```python
from build123d import *

# Parameters (mm, degrees)
SKETCH1_W               = 60
SKETCH1_H               = 160
BOSS_EXTRUDE1_DEPTH     = 3.175
M4_5_THROUGH_DEPTH      = 6.35
M4_5_THROUGH_DEPTH_BACK = 3.175
SKETCH3_R               = 2.75
SKETCH3_R_2             = 2.2
SKETCH4_R               = 1.3
M3_DRILL_DEPTH          = 8
SKETCH5_R               = 2.2
M4_THROUGH_DEPTH        = 6.35
SKETCH6_R               = 2.75
M5_THROUGH_DEPTH        = 6.35
SKETCH7_W               = 60
SKETCH7_H               = 30.2375
CUT_EXTRUDE1_DEPTH      = 6.35


with BuildPart() as part:
    # Sketch1 → Boss-Extrude1 (new, symmetric)
    with BuildSketch(Plane(origin=(0, 0, 0), x_dir=(1, 0, 0), z_dir=(0, 1, 0))):
        Rectangle(SKETCH1_W, SKETCH1_H)
    extrude(amount=BOSS_EXTRUDE1_DEPTH, both=True)

    # Sketch3 → M4/5_through (cut, two sides: drawn at the far end of the back side and taken through both)
    with BuildSketch(Plane(origin=(0, 0, 0), x_dir=(1, 0, 0), z_dir=(0, 1, 0)).offset(-M4_5_THROUGH_DEPTH_BACK)):
        with Locations(Location((20, 75.2375, 0), (0, 0, 270))):
            Circle(SKETCH3_R)
        with Locations(Location((20, 50.2375, 0), (0, 0, 270))):
            Circle(SKETCH3_R_2)
        with Locations(Location((-20, 50.2375, 0), (0, 0, 270))):
            Circle(SKETCH3_R_2)
        with Locations(Location((-20, 75.2375, 0), (0, 0, 270))):
            Circle(SKETCH3_R)
        with Locations(Location((0, 75.2375, 0), (0, 0, 270))):
            Circle(SKETCH3_R)
        with Locations(Location((0, 50.2375, 0), (0, 0, 270))):
            Circle(SKETCH3_R_2)
        with Locations(Location((20, -44.7625, 0), (0, 0, 270))):
            Circle(SKETCH3_R_2)
        with Locations(Location((-20, -44.7625, 0), (0, 0, 270))):
            Circle(SKETCH3_R_2)
        with Locations(Location((0, -44.7625, 0), (0, 0, 270))):
            Circle(SKETCH3_R_2)
    extrude(amount=M4_5_THROUGH_DEPTH + M4_5_THROUGH_DEPTH_BACK, mode=Mode.SUBTRACT)

    # Sketch4 → M3_DRILL (cut)
    with BuildSketch(Plane(origin=(0, 0, -80), x_dir=(-1, 0, 0), z_dir=(0, 0, -1))):
        with Locations((-12, 0)):
            Circle(SKETCH4_R)
        with Locations(Location((12, 0, 0), (0, 0, 180))):
            Circle(SKETCH4_R)
    extrude(amount=-M3_DRILL_DEPTH, mode=Mode.SUBTRACT)

    # Sketch5 → M4_through (cut)
    with BuildSketch(Plane(origin=(0, 3.175, 0), x_dir=(1, 0, 0), z_dir=(0, 1, 0))):
        with Locations(Location((-25.2375, -27.6625, 0), (0, 0, 270))):
            Circle(SKETCH5_R)
        with Locations(Location((25.2375, -27.6625, 0), (0, 0, 270))):
            Circle(SKETCH5_R)
        with Locations(Location((25.2375, 33.1375, 0), (0, 0, 270))):
            Circle(SKETCH5_R)
        with Locations(Location((-25.2375, 33.1375, 0), (0, 0, 270))):
            Circle(SKETCH5_R)
    extrude(amount=-M4_THROUGH_DEPTH, mode=Mode.SUBTRACT)

    # Sketch6 → M5_through (cut)
    with BuildSketch(Plane(origin=(0, 3.175, 0), x_dir=(1, 0, 0), z_dir=(0, 1, 0))):
        with Locations(Location((0, 16.2375, 0), (0, 0, 270))):
            Circle(SKETCH6_R)
        with Locations(Location((11.691342951, 9.4875, 0), (0, 0, 270))):
            Circle(SKETCH6_R)
        with Locations(Location((11.691342951, -4.0125, 0), (0, 0, 270))):
            Circle(SKETCH6_R)
        with Locations(Location((0, -10.7625, 0), (0, 0, 270))):
            Circle(SKETCH6_R)
        with Locations(Location((-11.691342951, -4.0125, 0), (0, 0, 270))):
            Circle(SKETCH6_R)
        with Locations(Location((-11.691342951, 9.4875, 0), (0, 0, 270))):
            Circle(SKETCH6_R)
    extrude(amount=-M5_THROUGH_DEPTH, mode=Mode.SUBTRACT)

    # Sketch7 → Cut-Extrude1 (cut)
    with BuildSketch(Plane(origin=(0, 3.175, 0), x_dir=(1, 0, 0), z_dir=(0, 1, 0))):
        with Locations((0, -64.88125)):
            Rectangle(SKETCH7_W, SKETCH7_H)
    extrude(amount=-CUT_EXTRUDE1_DEPTH, mode=Mode.SUBTRACT)


solid = part.part
```
Could you check a few things on this model? Use its own coordinates, in mm. A direction names the side the tool comes from. Round coordinates to 2 decimals unless told otherwise and drop trailing zeros. Loops run counter-clockwise (first coordinate to the right, second up) from the corner with the lowest first, then second, coordinate; pieces in that order, holes last. Notation, with made-up numbers: (71.5, 31) -> (110.5, 31) arc R17 ccw to (110.5, 60) -> close; hole circle Ø10 at (83, 71). An arc over 180 degrees is marked (long way). Put each result on its own line as item: value.
Q1. I want a section at B-B on x = 20. Write out the boundary of the cut face in (y, z) (1 decimal), and give its area (3 significant figures).
Checks:
outline: (-3.2, -80) -> (3.2, -80) -> (3.2, -78) -> (-3.2, -78) -> close; (-3.2, -72.5) -> (3.2, -72.5) -> (3.2, -52.4) -> (-3.2, -52.4) -> close; (-3.2, -48) -> (3.2, -48) -> (3.2, 42.6) -> (-3.2, 42.6) -> close; (-3.2, 47) -> (3.2, 47) -> (3.2, 49.8) -> (-3.2, 49.8) -> close
area: 733 mm2
Q2. For pin 1 Ø5 at (x, z) = (-20, -75.24) entering from +Y, with a flat end and sliding along its axis, tell me the tip position at first contact or that it passes through.
Checks:
pin 1: through
Q3. Thinking about a two-plate mould opening in X: for faces 1 (the flat face through (-7, -3.175, -16)), 2 (the cylindrical face through (-20.843, -0.044, 46.795)), 3 (the flat face through (30, 0, -14)), 4 (the cylindrical face through (-0.843, -0.044, -48.205)), which applies, pulls with the +X half, pulls with the -X half, needs draft (parallel to the pull), parting line crosses it, or undercut?
Checks:
face 1: needs draft
face 2: undercut
face 3: pulls with the +X half
face 4: undercut
Q4. I want a section at C-C on y = 0. Give the number of separate pieces and of enclosed holes in the cut face, and give its area (3 significant figures).
Checks:
separate pieces: 1
enclosed holes: 19
area: 7,380 mm2
Q5. Please list where these lines run through material, in increasing order: line 1 (Z direction, x = 20, y = 1.5); line 2 (Z direction, x = 25, y = 0.75); line 3 (Z direction, x = 12, y = 0.25). Write a range as from..to.
Checks:
line 1: -80..-77.99, -72.49..-52.44, -48.04..42.56, 46.96..49.76
line 2: -80..-35.32, -30.95..25.48, 29.85..49.76
line 3: -72..-12.22, -6.75..1.28, 6.75..49.76
Q6. Which directions (+Z, -Z, +X, -X, +Y, -Y) give clear straight access to the entire face, cutting with the end or side of a thin tool? Please do faces 5 (the flat face through (12, 0, -72)), 6 (the cylindrical face through (-20.843, -0.044, -48.205)).
Checks:
face 5: -Z
face 6: +Y, -Y
Q7. I want a section at A-A on x = 0. Write out the boundary of the cut face in (y, z) (1 decimal), and give its area (3 significant figures).
Checks:
outline: (-3.2, -80) -> (3.2, -80) -> (3.2, -78) -> (-3.2, -78) -> close; (-3.2, -72.5) -> (3.2, -72.5) -> (3.2, -52.4) -> (-3.2, -52.4) -> close; (-3.2, -48) -> (3.2, -48) -> (3.2, -19) -> (-3.2, -19) -> close; (-3.2, -13.5) -> (3.2, -13.5) -> (3.2, 8) -> (-3.2, 8) -> close; (-3.2, 13.5) -> (3.2, 13.5) -> (3.2, 42.6) -> (-3.2, 42.6) -> close; (-3.2, 47) -> (3.2, 47) -> (3.2, 49.8) -> (-3.2, 49.8) -> close
area: 663 mm2
Q8. I want a section at D-D on z = 10. Write out the boundary of the cut face in (x, y) (3 decimals), and give its area (3 significant figures).
Checks:
outline: (-30, -3.175) -> (-2.642, -3.175) -> (-2.642, 3.175) -> (-30, 3.175) -> close; (2.642, -3.175) -> (30, -3.175) -> (30, 3.175) -> (2.642, 3.175) -> close
area: 347 mm2
